Design review of the part built by this model. Coordinates are the model's own, in mm. A direction names the side the tool comes from. Round coordinates to 2 decimals unless told otherwise and drop trailing zeros. Order: outer loops, then holes, each group sorted by start corner. A loop starts at its lowest first (then second) coordinate and runs counter-clockwise, first axis right, second up. Notation, with made-up numbers: (16.5, 79) - (33.5, 79) arc R33 ccw to (33.5, 113) - close; hole circle Ø10 at (19.25, 48.5). An arc over 180 degrees is marked (long way). Use CSV: the item, a comma, the result in double quotes.
from build123d import *

# Parameters (mm, degrees)
F0_R     = 7.9375
F1_DEPTH = 19.05


# Not quite as in the source:
# - a feature of the source that left no trace in its solid (it failed there, or was rolled back) is left out


with BuildPart() as f1:
    # F0 (on Top) → F1 (new body)
    with BuildSketch(Plane.XY):
        with BuildLine():
            ThreePointArc((-253.1241280528, -50.8), (-238.245152537, -14.8789755157), (-202.3241280528, 0))
            Line((-202.3241280528, 0), (-303.9241280528, 0))
            Line((-303.9241280528, 0), (-303.9241280528, -50.8))
            Line((-303.9241280528, -50.8), (-253.1241280528, -50.8))
        make_face()
        with BuildLine():
            ThreePointArc((-151.5241280528, -50.8), (-166.4031035685, -14.8789755157), (-202.3241280528, 0))
            ThreePointArc((-202.3241280528, 0), (-238.245152537, -14.8789755157), (-253.1241280528, -50.8))
            Line((-253.1241280528, -50.8), (-151.5241280528, -50.8))
        make_face()
        with BuildLine():
            Line((-100.7241280528, -50.8), (-100.7241280528, 0))
            Line((-100.7241280528, 0), (-202.3241280528, 0))
            ThreePointArc((-202.3241280528, 0), (-166.4031035685, -14.8789755157), (-151.5241280528, -50.8))
            Line((-151.5241280528, -50.8), (-100.7241280528, -50.8))
        make_face()
        with BuildLine():
            ThreePointArc((-253.1241280528, -50.8), (-202.3241280528, -101.6), (-151.5241280528, -50.8))
            Line((-151.5241280528, -50.8), (-253.1241280528, -50.8))
        make_face()
        with Locations((-202.3241280528, -75.8825)):
            Circle(F0_R, mode=Mode.SUBTRACT)
    extrude(amount=F1_DEPTH)


solid = f1.part
1) For faces 4 (the face through (-203.441, -101.588, 9.392)), 5 (the face through (-279, -50.8, 9)), list the 3-axis set-ups (+Z, -Z, +X, -X, +Y, -Y) from which the entire face can be reached by the end or side of a thin tool; tool diameter is ignored.
Data:
face 4,"+Z, -Z, -Y"
face 5,"+Z, -Z, -X, -Y"
2) Insertion check: pin 1 Ø4 at (x, z) = (-214.5, 12) entering from -Y; pin 2 Ø12.5 at (x, y) = (-202.32, -75.88) entering from +Z. Each pin has a flat end and moves straight along its axis. Give the tip position at first contact, or say it passes through.
Data:
pin 1,"stops at y = -100.57"
pin 2,"passes through"
3) The part is to be moulded in two halves that separate along Y. For faces 1 (the face through (-126, -50.8, 9)), 2 (the face through (-100.724, -26, 9)), 3 (the face through (-194.99, -78.92, 9.39)), say which applies: +Y half, -Y half, draft (parallel to the pull), parting line (faces both ways), or undercut.
Data:
face 1,"-Y half"
face 2,"draft"
face 3,"undercut"
4) We need section C-C (y = -61.5). Give the boundary of the cut face in (x, z).
Data:
outline,"(-251.98, 0) - (-152.66, 0) - (-152.66, 19.05) - (-251.98, 19.05) - close"
5) To check wall thickness, follow L1, parallel to Y at x = -270.5, z = 10; L2, parallel to Y at x = -196, z = 14.25; L3, parallel to X at y = -73.5, z = 3.5. State the ranges of each line that lie inside material, in increasing order. Write a range as from..to.
Data:
L1,"y = -50.8..0"
L2,"y = -101.2..-80.68, -71.09..0"
L3,"x = -247.77..-209.9, -194.75..-156.88"
6) We need section B-B (x = -263). Give the boundary of the cut face in (y, z).
Data:
outline,"(-50.8, 0) - (0, 0) - (0, 19.05) - (-50.8, 19.05) - close"
7) We need section A-A (z = 10.25). Give the boundary of the cut face in (x, y) (1 decimal), then the cut area to 3 significant figures.
Data:
outline,"(-303.9, -50.8) - (-253.1, -50.8) arc R50.8 ccw to (-151.5, -50.8) - (-100.7, -50.8) - (-100.7, 0) - (-303.9, 0) - close; hole circle Ø15.9 at (-202.3, -75.9)"
area,"14,200 mm2"
